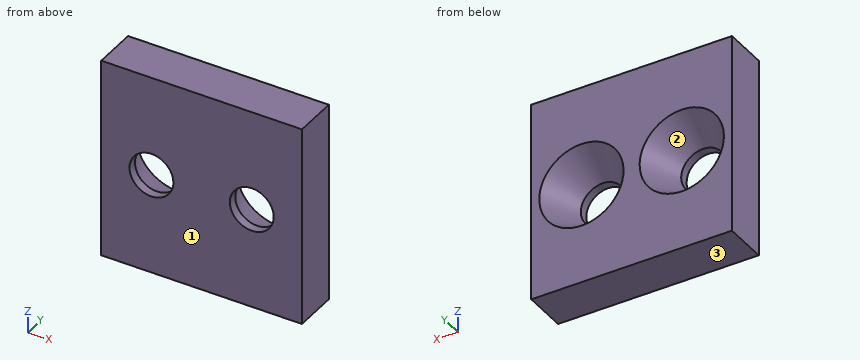
```python
from build123d import *

# Parameters (mm, degrees)
SKETCH1_W                    = 32
SKETCH1_H                    = 32
BOSS_EXTRUDE1_DEPTH          = 7
CSK_FOR_M6_SFHCS1_AT_2_COUNT = 2
CSK_FOR_M6_SFHCS1_AT_2_PITCH = 16


with BuildPart() as part:
    # Sketch1 → Boss-Extrude1 (new body)
    with BuildSketch(Plane(origin=(0, 0, 0), x_dir=(1, 0, 0), z_dir=(0, 1, 0))):
        with Locations((16, 16)):
            Rectangle(SKETCH1_W, SKETCH1_H)
    extrude(amount=BOSS_EXTRUDE1_DEPTH)

    # Sketch4 → CSK for M6 SFHCS1 (revolve, cut)
    with BuildSketch(Plane(origin=(8, 7, -16), x_dir=(0, 0, 1), z_dir=(1, 0, 0))):
        Polygon((0, 0), (0, 7), (3.5, 7), (3.5, 5.5772036), (6.72, 0), align=None)
    csk_for_m6_sfhcs1 = revolve(axis=Axis((8, 13.35, -16), (0, -1, 0)), mode=Mode.SUBTRACT)

    # CSK for M6 SFHCS1 at 2: CSK for M6 SFHCS1 ×2
    with Locations(*[(i * CSK_FOR_M6_SFHCS1_AT_2_PITCH, 0, 0) for i in range(1, CSK_FOR_M6_SFHCS1_AT_2_COUNT)]):
        add(csk_for_m6_sfhcs1, mode=Mode.SUBTRACT)


solid = part.part
```
Geometry check sheet. Reference: the model listing, model coordinates, mm. Face numbers are marked on the shaded views. Give positions to 0.01 mm unless a question says otherwise; leave off trailing zeros. Order: outer loops, then holes, each group sorted by start corner. A loop starts at its lowest first (then second) coordinate and runs counter-clockwise, first axis right, second up. Notation, with made-up numbers: (1, 64) - (43, 64) arc R33 cw to (43, 93) - close; hole circle Ø1 at (-9, -2). An arc over 180 degrees is marked (long way). Write item = value, one per line. Start each with the question number.
1) Section check A-A (x = 24). Enter the section's corners in (y, z), then the cut area to 3 significant figures.
2) Draft check along Z on the marked faces 1, 2 and 3. Enter one of: released by +Z, released by -Z, zero draft, split by the parting line, or undercut.
3) Scan lines: L1, parallel to X at y = 1.15, z = -16; L2, parallel to Z at x = 24, y = 0.5; L3, parallel to X at y = 2.5, z = -15.5. Record each from-to range of solid material in increasing order.
4) Gauge pin test, flat end, axial feed: pin 1 Ø8 at (x, z) = (8, -16) entering from -Y. Record the tip position at first contact, or that the pin passes through.
5) Section check D-D (y = 4). Enter the section's corners in (x, z).
6) Section check B-B (z = -16). Enter the section's corners in (x, y), then the cut area to 3 significant figures.
7) Section check C-C (y = 0.5). Enter the section's corners in (x, z), then the cut area to 3 significant figures.
Geometry check:
q1.outline = (0, -32) - (7, -32) - (7, -22.72) - (1.42, -19.5) - (0, -19.5) - close; (0, -12.5) - (1.42, -12.5) - (7, -9.28) - (7, 0) - (0, 0) - close
q1.area = 157 mm2
q2.face_1 = zero draft
q2.face_2 = undercut
q2.face_3 = released by -Z
q3.L1 = 0 to 4.5, 11.5 to 20.5, 27.5 to 32
q3.L2 = -32 to -19.5, -12.5 to 0
q3.L3 = 0 to 3.91, 12.09 to 19.91, 28.09 to 32
q4.pin_1 = 0
q5.outline = (0, -32) - (32, -32) - (32, 0) - (0, 0) - close; hole circle Ø9.98 at (8, -16); hole circle Ø9.98 at (24, -16)
q6.outline = (0, 0) - (4.5, 0) - (4.5, 1.42) - (1.28, 7) - (0, 7) - close; (11.5, 0) - (20.5, 0) - (20.5, 1.42) - (17.28, 7) - (14.72, 7) - (11.5, 1.42) - close; (27.5, 0) - (32, 0) - (32, 7) - (30.72, 7) - (27.5, 1.42) - close
q6.area = 90.1 mm2
q7.outline = (0, -32) - (32, -32) - (32, 0) - (0, 0) - close; hole circle Ø7 at (8, -16); hole circle Ø7 at (24, -16)
q7.area = 947 mm2
